```python
from build123d import *

# Parameters (mm, degrees)
SKETCH1_W                      = 100
SKETCH1_H                      = 100
SKETCH1_W_2                    = 94
SKETCH1_H_2                    = 94
EXTRUDE_THIN1_DEPTH            = 130
FILLET1_R                      = 0.5
FILLET2_R                      = 3
F_8_0_8_DIAMETER_HOLE2_D       = 8
F_8_0_8_DIAMETER_HOLE3_D       = 8
F_10_0_10_DIAMETER_HOLE1_D     = 10
F_10_0_10_DIAMETER_HOLE2_D     = 10
F_6_0_6_DIAMETER_HOLE2_D       = 6
F_6_0_6_DIAMETER_HOLE2_DEPTH   = 3
F_6_0_6_DIAMETER_HOLE3_D       = 6
F_6_0_6_DIAMETER_HOLE3_DEPTH   = 3
F_21_0_21_DIAMETER_HOLE1_D     = 21
F_21_0_21_DIAMETER_HOLE1_DEPTH = 3
F_6_0_6_DIAMETER_HOLE1_D       = 6
F_6_0_6_DIAMETER_HOLE1_DEPTH   = 3
CUT_EXTRUDE1_REACH             = 173.464
SKETCH27_R                     = 2
SKETCH27_R_2                   = 3.5
CUT_EXTRUDE2_REACH             = 173.464
SKETCH31_R                     = 4


with BuildPart() as part:
    # Sketch1 → Extrude-Thin1 (new body)
    with BuildSketch(Plane.XY):
        Rectangle(SKETCH1_W, SKETCH1_H)
        Rectangle(SKETCH1_W_2, SKETCH1_H_2, mode=Mode.SUBTRACT)
    extrude(amount=EXTRUDE_THIN1_DEPTH)

    # Fillet1
    fillet1_edges = [part.edges().sort_by_distance(p)[0] for p in [
        (47, -47, 65),
        (47, 47, 65),
        (-47, 47, 65),
        (-47, -47, 65),
    ]]
    fillet(fillet1_edges, radius=FILLET1_R)

    # Fillet2
    fillet2_edges = [part.edges().sort_by_distance(p)[0] for p in [
        (50, -50, 65),
        (-50, -50, 65),
        (-50, 50, 65),
        (50, 50, 65),
    ]]
    fillet(fillet2_edges, radius=FILLET2_R)

    # Ø8.0 (8) Diameter Hole2 (through all)
    with Locations(Plane(origin=(0, 50, 0), x_dir=(1, 0, 0), z_dir=(0, 1, 0))):
        with Locations((28, -32), (28, -90)):
            Hole(F_8_0_8_DIAMETER_HOLE2_D / 2)

    # Ø8.0 (8) Diameter Hole3 (through all)
    with Locations(Plane(origin=(50, 0, 0), x_dir=(0, 0, -1), z_dir=(1, 0, 0))):
        with Locations((-14, 31), (-116, 31)):
            Hole(F_8_0_8_DIAMETER_HOLE3_D / 2)

    # Ø10.0 (10) Diameter Hole1 (through all)
    with Locations(Plane(origin=(0, 50, 0), x_dir=(1, 0, 0), z_dir=(0, 1, 0))):
        with Locations((-34, -56)):
            Hole(F_10_0_10_DIAMETER_HOLE1_D / 2)

    # Ø10.0 (10) Diameter Hole2 (through all)
    with Locations(Plane(origin=(50, 0, 0), x_dir=(0, 0, -1), z_dir=(1, 0, 0))):
        with Locations((-44, -31)):
            Hole(F_10_0_10_DIAMETER_HOLE2_D / 2)

    # Ø6.0 (6) Diameter Hole2
    with Locations(Plane.ZY.offset(50)):
        with Locations((56, -15), (56, 35)):
            Hole(F_6_0_6_DIAMETER_HOLE2_D / 2, depth=F_6_0_6_DIAMETER_HOLE2_DEPTH)

    # Ø6.0 (6) Diameter Hole3
    with Locations(Plane(origin=(0, -50, 0), x_dir=(-1, 0, 0), z_dir=(0, -1, 0))):
        with Locations((20, -44), (-35, -44)):
            Hole(F_6_0_6_DIAMETER_HOLE3_D / 2, depth=F_6_0_6_DIAMETER_HOLE3_DEPTH)

    # Ø21.0 (21) Diameter Hole1
    with Locations(Plane(origin=(50, 0, 0), x_dir=(0, 0, -1), z_dir=(1, 0, 0))):
        with Locations((-70, 0)):
            Hole(F_21_0_21_DIAMETER_HOLE1_D / 2, depth=F_21_0_21_DIAMETER_HOLE1_DEPTH)

    # Ø6.0 (6) Diameter Hole1
    with Locations(Plane(origin=(50, 0, 0), x_dir=(0, 0, -1), z_dir=(1, 0, 0))):
        with Locations((-41.157258279, -16.652364697), (-53.347635303, 28.842741721), (-98.842741721, 16.652364697), (-86.652364697, -28.842741721)):
            Hole(F_6_0_6_DIAMETER_HOLE1_D / 2, depth=F_6_0_6_DIAMETER_HOLE1_DEPTH)

    # Sketch27 → Cut-Extrude1 (cut, up to next)
    with BuildSketch(Plane(origin=(50, 0, 0), x_dir=(0, 0, -1), z_dir=(1, 0, 0)), mode=Mode.PRIVATE) as cut_extrude1_sk1:
        with Locations(Location((-5, 13, 0), (0, 0, 90))):
            Circle(SKETCH27_R)
    cut_extrude1_tool1 = extrude(cut_extrude1_sk1.sketch, amount=-CUT_EXTRUDE1_REACH, mode=Mode.PRIVATE) & part.part
    # Sketch27 → Cut-Extrude1 (cut, up to next)
    with BuildSketch(Plane(origin=(50, 0, 0), x_dir=(0, 0, -1), z_dir=(1, 0, 0)), mode=Mode.PRIVATE) as cut_extrude1_sk2:
        with Locations(Location((-5, 4, 0), (0, 0, 90))):
            Circle(SKETCH27_R)
    cut_extrude1_tool2 = extrude(cut_extrude1_sk2.sketch, amount=-CUT_EXTRUDE1_REACH, mode=Mode.PRIVATE) & part.part
    # Sketch27 → Cut-Extrude1 (cut, up to next)
    with BuildSketch(Plane(origin=(50, 0, 0), x_dir=(0, 0, -1), z_dir=(1, 0, 0)), mode=Mode.PRIVATE) as cut_extrude1_sk3:
        with Locations(Location((-23, 8.5, 0), (0, 0, 90))):
            Circle(SKETCH27_R_2)
    cut_extrude1_tool3 = extrude(cut_extrude1_sk3.sketch, amount=-CUT_EXTRUDE1_REACH, mode=Mode.PRIVATE) & part.part
    # Sketch27 → Cut-Extrude1 (cut, up to next)
    with BuildSketch(Plane(origin=(50, 0, 0), x_dir=(0, 0, -1), z_dir=(1, 0, 0)), mode=Mode.PRIVATE) as cut_extrude1_sk4:
        with Locations(Location((-107, 8.5, 0), (0, 0, 270))):
            Circle(SKETCH27_R_2)
    cut_extrude1_tool4 = extrude(cut_extrude1_sk4.sketch, amount=-CUT_EXTRUDE1_REACH, mode=Mode.PRIVATE) & part.part
    # Sketch27 → Cut-Extrude1 (cut, up to next)
    with BuildSketch(Plane(origin=(50, 0, 0), x_dir=(0, 0, -1), z_dir=(1, 0, 0)), mode=Mode.PRIVATE) as cut_extrude1_sk5:
        with Locations(Location((-125, 4, 0), (0, 0, 270))):
            Circle(SKETCH27_R)
    cut_extrude1_tool5 = extrude(cut_extrude1_sk5.sketch, amount=-CUT_EXTRUDE1_REACH, mode=Mode.PRIVATE) & part.part
    # Sketch27 → Cut-Extrude1 (cut, up to next)
    with BuildSketch(Plane(origin=(50, 0, 0), x_dir=(0, 0, -1), z_dir=(1, 0, 0)), mode=Mode.PRIVATE) as cut_extrude1_sk6:
        with Locations(Location((-125, 13, 0), (0, 0, 270))):
            Circle(SKETCH27_R)
    cut_extrude1_tool6 = extrude(cut_extrude1_sk6.sketch, amount=-CUT_EXTRUDE1_REACH, mode=Mode.PRIVATE) & part.part
    add(cut_extrude1_tool1.solids().sort_by_distance((50, 13, 5))[0], mode=Mode.SUBTRACT)
    add(cut_extrude1_tool2.solids().sort_by_distance((50, 4, 5))[0], mode=Mode.SUBTRACT)
    add(cut_extrude1_tool3.solids().sort_by_distance((50, 8.5, 23))[0], mode=Mode.SUBTRACT)
    add(cut_extrude1_tool4.solids().sort_by_distance((50, 8.5, 107))[0], mode=Mode.SUBTRACT)
    add(cut_extrude1_tool5.solids().sort_by_distance((50, 4, 125))[0], mode=Mode.SUBTRACT)
    add(cut_extrude1_tool6.solids().sort_by_distance((50, 13, 125))[0], mode=Mode.SUBTRACT)

    # Sketch31 → Cut-Extrude2 (cut, up to next)
    with BuildSketch(Plane.ZY.offset(50), mode=Mode.PRIVATE) as cut_extrude2_sk1:
        with Locations(Location((14, -37, 0), (0, 0, 270))):
            Circle(SKETCH31_R)
    cut_extrude2_tool1 = extrude(cut_extrude2_sk1.sketch, amount=-CUT_EXTRUDE2_REACH, mode=Mode.PRIVATE) & part.part
    # Sketch31 → Cut-Extrude2 (cut, up to next)
    with BuildSketch(Plane.ZY.offset(50), mode=Mode.PRIVATE) as cut_extrude2_sk2:
        with Locations(Location((110, -37, 0), (0, 0, 270))):
            Circle(SKETCH31_R)
    cut_extrude2_tool2 = extrude(cut_extrude2_sk2.sketch, amount=-CUT_EXTRUDE2_REACH, mode=Mode.PRIVATE) & part.part
    add(cut_extrude2_tool1.solids().sort_by_distance((-50, -37, 14))[0], mode=Mode.SUBTRACT)
    add(cut_extrude2_tool2.solids().sort_by_distance((-50, -37, 110))[0], mode=Mode.SUBTRACT)


solid = part.part
```
Input: part model. Units: mm. Frame: model coordinates. A direction names the side the tool comes from. Round coordinates to 2 decimals unless told otherwise and drop trailing zeros. Loops run counter-clockwise (first coordinate to the right, second up) from the corner with the lowest first, then second, coordinate; pieces in that order, holes last. Notation, with made-up numbers: (-20.5, 82) - (30.5, 82) arc R12 ccw to (30.5, 90) - close; hole circle Ø2 at (1, 85.5). An arc over 180 degrees is marked (long way). One line per item, written item: value. Start each with the question number.
(1) Section D-D, the plane x = 15. Return loops of the section in (y, z), plus the area to 3 significant figures.
(2) Contact query for flat-ended pins moving along their axis: P1, Ø6.5, axis at y = 31, z = 116, coming from the -X side; P2, Ø5, axis at x = 35, z = 44, coming from the -Y side; P3, Ø4, axis at y = -3.5, z = 73.5, coming from the +X side. Output: stop coordinate, or through.
(3) Section C-C, the plane z = 14. Return loops of the section in (x, y), plus the area to 3 significant figures.
(4) Access query for faces 4 (the flat face through (-47, -1, 64)), 5 (the cylindrical face through (-49, -31, 39)), 6 (the cylindrical face through (48.48, 0.46, 59.51)), 7 (the cylindrical face through (32.79, -48.48, 41.97)), 8 (the cylindrical face through (-48.521, -36.479, 113.966)). Directions: +Z, -Z, +X, -X, +Y, -Y. A direction counts if a zero-diameter tool reaches every point of the face in a straight line with its end or side. Return the directions, or none.
(5) Section A-A, the plane z = 125. Return loops of the section in (x, y).
(6) Section B-B, the plane x = 28. Return loops of the section in (y, z), plus the area to 3 significant figures.
(7) Draft query along Z for faces 1 (the cylindrical face through (48.479, 32.201, 119.815)), 2 (the flat face through (-4, -48, 0)), 3 (the flat face through (50, -11, 64)). Return one class per face: +Z half, -Z half, draft (parallel to the pull), parting line (faces both ways), or undercut.
(8) Ray query, line 1 (Y direction, x = 4, z = 97.5); line 2 (Z direction, x = 48, y = 8.5). Return the intervals inside material, ascending. Write a range as [from, to].
Results below:
1. outline: (-50, 0) - (-47, 0) - (-47, 130) - (-50, 130) - close; (47, 0) - (50, 0) - (50, 130) - (47, 130) - close
1. area: 780 mm^2
2. P1: through
2. P2: y = 47
2. P3: x = -47
3. outline: (-50, -47) arc R3 ccw to (-47, -50) - (47, -50) arc R3 ccw to (50, -47) - (50, 27) - (47, 27) - (47, -46.5) arc R0.5 cw to (46.5, -47) - (-46.5, -47) arc R0.5 cw to (-47, -46.5) - (-47, -41) - (-50, -41) - close; (-50, -33) - (-47, -33) - (-47, 27) - (-50, 27) - close; (-50, 35) - (-47, 35) - (-47, 46.5) arc R0.5 cw to (-46.5, 47) - (46.5, 47) arc R0.5 cw to (47, 46.5) - (47, 35) - (50, 35) - (50, 47) arc R3 ccw to (47, 50) - (-47, 50) arc R3 ccw to (-50, 47) - close
3. area: 1,080 mm^2
4. face 4: +Z, -Z
4. face 5: +X, -X
4. face 6: +X
4. face 7: -Y
4. face 8: -X
5. outline: (-50, -47) arc R3 ccw to (-47, -50) - (47, -50) arc R3 ccw to (50, -47) - (50, 2) - (47, 2) - (47, -46.5) arc R0.5 cw to (46.5, -47) - (-46.5, -47) arc R0.5 cw to (-47, -46.5) - (-47, 46.5) arc R0.5 cw to (-46.5, 47) - (46.5, 47) arc R0.5 cw to (47, 46.5) - (47, 15) - (50, 15) - (50, 47) arc R3 ccw to (47, 50) - (-47, 50) arc R3 ccw to (-50, 47) - close; (47, 6) - (50, 6) - (50, 11) - (47, 11) - close
6. outline: (-50, 0) - (-47, 0) - (-47, 28) - (-50, 28) - close; (-50, 36) - (-47, 36) - (-47, 86) - (-50, 86) - close; (-50, 94) - (-47, 94) - (-47, 130) - (-50, 130) - close; (47, 0) - (50, 0) - (50, 28) - (47, 28) - close; (47, 36) - (50, 36) - (50, 86) - (47, 86) - close; (47, 94) - (50, 94) - (50, 130) - (47, 130) - close
6. area: 684 mm^2
7. face 1: undercut
7. face 2: -Z half
7. face 3: draft
8. line 1: [-50, -47], [47, 50]
8. line 2: [0, 19.5], [26.5, 63.84], [76.16, 103.5], [110.5, 130]
